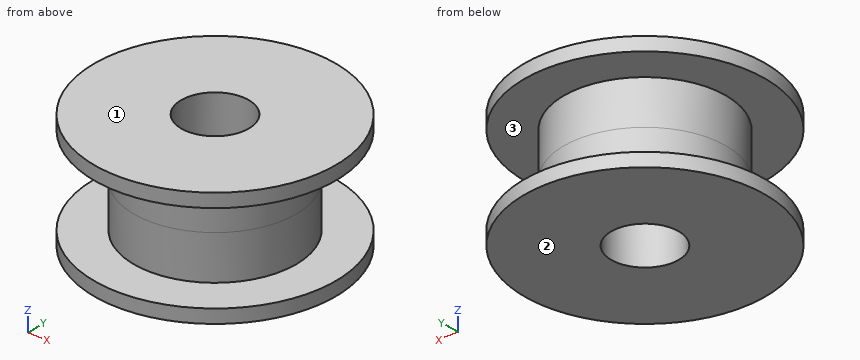
from build123d import *

# Parameters (mm, degrees)
SKETCH6_R           = 6
BOSS_EXTRUDE1_DEPTH = 3.25
SKETCH8_R           = 8.925
BOSS_EXTRUDE2_DEPTH = 1
SKETCH9_R           = 2.5
CUT_EXTRUDE1_DEPTH  = 14.318173674


with BuildPart() as part:
    # Sketch6 → Boss-Extrude1 (new body)
    with BuildSketch(Plane.XY):
        with Locations(Location((0, 0, 0), (0, 0, 180))):
            Circle(SKETCH6_R)
    boss_extrude1 = extrude(amount=BOSS_EXTRUDE1_DEPTH)

    # Sketch8 → Boss-Extrude2 (add)
    with BuildSketch(Plane(origin=(0, 0, 0), x_dir=(-1, 0, 0), z_dir=(0, 0, -1))):
        Circle(SKETCH8_R)
    boss_extrude2 = extrude(amount=BOSS_EXTRUDE2_DEPTH)

    # Sketch9 → Cut-Extrude1 (cut, through all)
    with BuildSketch(Plane(origin=(0, 0, -1), x_dir=(-1, 0, 0), z_dir=(0, 0, -1))):
        Circle(SKETCH9_R)
    cut_extrude1 = extrude(amount=-CUT_EXTRUDE1_DEPTH, mode=Mode.SUBTRACT)

    # Mirror2: Boss-Extrude1, Boss-Extrude2, Cut-Extrude1 across plane
    add(boss_extrude1.mirror(Plane.XY.offset(3.25)))
    add(boss_extrude2.mirror(Plane.XY.offset(3.25)))
    add(cut_extrude1.mirror(Plane.XY.offset(3.25)), mode=Mode.SUBTRACT)


solid = part.part
For this review, take the finished solid that the model builds, in its own axes (mm). Face numbers are marked on the shaded views. Round coordinates to 2 decimals unless told otherwise and drop trailing zeros. Loops run counter-clockwise (first coordinate to the right, second up) from the corner with the lowest first, then second, coordinate; pieces in that order, holes last. Notation, with made-up numbers: (23, 28.25) - (62, 28.25) arc R20 cw to (62, 40.25) - close; hole circle Ø9 at (40.25, 26). An arc over 180 degrees is marked (long way). One line per item, written item: value. Start each with the question number.
Item 1: The part is to be moulded in two halves that separate along Z. For the marked faces 1, 2 and 3, say which applies: +Z half, -Z half, draft (parallel to the pull), parting line (faces both ways), or undercut.
Item 2: Take a section at C-C (z = 0.25). Give the boundary of the cut face in (x, y).
Item 3: Take a section at A-A (y = 0). Give the boundary of the cut face in (x, z) (3 decimals).
Item 4: Take a section at D-D (x = 6.75). Give the boundary of the cut face in (y, z), plus the area to 3 significant figures.
Item 5: Clearance check with flat-ended pins moving along their axes: pin 1 Ø1.5 at (y, z) = (2.5, 3.5) entering from -X; pin 2 Ø4 at (x, z) = (-3, 4) entering from -Y; pin 3 Ø6 at (x, y) = (0, 0) entering from -Z; pin 4 Ø4 at (x, z) = (-4, 3.5) entering from -Y. State where each tip first meets the part, or that it passes through.
Item 6: For L1, parallel to Y at x = 0, z = 5.3; L2, parallel to Z at x = -4.25, y = -7.25; L3, parallel to Y at x = 0.75, z = 5.75, list the stretches that pass through material, from the lowest coordinate up.
Answer below:
1. face 1: +Z half
1. face 2: -Z half
1. face 3: undercut
2. outline: circle Ø12 at (0, 0); hole circle Ø5 at (0, 0)
3. outline: (-8.925, -1) - (-2.5, -1) - (-2.5, 7.5) - (-8.925, 7.5) - (-8.925, 6.5) - (-6, 6.5) - (-6, 0) - (-8.925, 0) - close; (2.5, -1) - (8.925, -1) - (8.925, 0) - (6, 0) - (6, 6.5) - (8.925, 6.5) - (8.925, 7.5) - (2.5, 7.5) - close
4. outline: (-5.84, -1) - (5.84, -1) - (5.84, 0) - (-5.84, 0) - close; (-5.84, 6.5) - (5.84, 6.5) - (5.84, 7.5) - (-5.84, 7.5) - close
4. area: 23.4 mm2
5. pin 1: stops at x = -5.74
5. pin 2: stops at y = -5.92
5. pin 3: stops at z = -1
5. pin 4: stops at y = -5.66
6. L1: y = -6 to -2.5, 2.5 to 6
6. L2: z = -1 to 0, 6.5 to 7.5
6. L3: y = -5.95 to -2.38, 2.38 to 5.95
